Build history of the part. All positions in model axes, mm. A direction names the side the tool comes from. Round coordinates to 2 decimals unless told otherwise and drop trailing zeros. Write each loop counter-clockwise with the first axis right and the second up, starting at its lowest first coordinate (ties: lowest second). Pieces come first, ordered by that corner, then holes.
1) Saw through at B-B (x = -6.35). Write the cut outline in (y, z), plus the area to 3 significant figures.
2) Wall check: probe 1 along Z at (x, y) = (-6, 4); probe 2 along Z at (x, y) = (-33.76, 4); probe 3 along X at (y, z) = (5.5, -13.41). Give the ranges that are in metal, low to high.
3) Saw through at C-C (y = 25). Write the cut outline in (x, z).
4) Flat gauge pins, fed straight in: pin 1 (2 mm diameter, centred on y = 33, z = -23.5, fed in from +X); pin 2 (12 mm diameter, centred on x = -30.5, z = 23, fed in from +Y); pin 3 (1.5 mm diameter, centred on x = 29.5, y = 32, fed in from +Z). Where does each tip first touch, or does it go through?
5) Which spindle directions (+Z, -Z, +X, -X, +Y, -Y) get a long thin tool onto all of the face, cutting with end or side? Do faces 5 (the flat face through (-59, 6, 25.4)), 6 (the flat face through (12.986, 18, 0)), 7 (the flat face through (14.986, 23, 0)), 8 (the flat face through (14.986, 32, 23)). Say none if no direction does.
6) Saw through at A-A (z = 0). Write the cut outline in (x, y).
7) Pull direction X, two halves, no side cores. Call faces 1 (the cylindrical face through (-6.61, 3.5, -65.085)), 2 (the flat face through (51, 18, 25.4)), 3 (the flat face through (-20, 7.1, -1)), 4 (the flat face through (86.36, 23, 0)): +X half, -X half, draft (parallel to the pull), parting line (faces both ways), or undercut.
8) Saw through at D-D (x = 49). Write the cut outline in (y, z), plus the area to 3 significant figures.
from build123d import *

# Parameters (mm, degrees)
SKETCH1_W           = 172.72
SKETCH1_H           = 50.8
BOSS_EXTRUDE1_DEPTH = 12.7
BOSS_EXTRUDE2_DEPTH = 71.374
SKETCH5_W           = 50.8
SKETCH5_H           = 27.94
BOSS_EXTRUDE3_DEPTH = 2
SKETCH6_W           = 50.8
SKETCH6_H           = 15.24
BOSS_EXTRUDE4_DEPTH = 2
CUT_EXTRUDE1_DEPTH  = 51.8
FILLET1_R           = 1
SKETCH8_R           = 12.7
CUT_EXTRUDE2_DEPTH  = 7.1
SKETCH9_R           = 5.9563
BOSS_EXTRUDE5_DEPTH = 7.1
SKETCH10_R          = 1.5
CUT_EXTRUDE3_DEPTH  = 7.1


with BuildPart() as part:
    # Sketch1 → Boss-Extrude1 (new body)
    with BuildSketch(Plane(origin=(0, 0, 0), x_dir=(1, 0, 0), z_dir=(0, 1, 0))):
        Rectangle(SKETCH1_W, SKETCH1_H)
    extrude(amount=BOSS_EXTRUDE1_DEPTH)

    # Sketch4 → Boss-Extrude2 (add)
    with BuildSketch(Plane(origin=(86.36, 0, 0), x_dir=(0, 0, -1), z_dir=(1, 0, 0))):
        with BuildLine():
            Line((-25.4, 12.7), (-25.4, 35.8))
            Line((-25.4, 35.8), (-20.1, 35.8))
            ThreePointArc((-20.1, 35.8), (0, 15.7), (20.1, 35.8))
            Line((20.1, 35.8), (25.4, 35.8))
            Line((25.4, 35.8), (25.4, 12.7))
            Line((25.4, 12.7), (-25.4, 12.7))
        make_face()
    extrude(amount=-BOSS_EXTRUDE2_DEPTH)

    # Sketch5 → Boss-Extrude3 (add)
    with BuildSketch(Plane(origin=(86.36, 0, 0), x_dir=(0, 0, -1), z_dir=(1, 0, 0))):
        with Locations((0, 13.97)):
            Rectangle(SKETCH5_W, SKETCH5_H)
    extrude(amount=BOSS_EXTRUDE3_DEPTH)

    # Sketch6 → Boss-Extrude4 (add)
    with BuildSketch(Plane.ZY.offset(-14.986)):
        with Locations((0, 20.32)):
            Rectangle(SKETCH6_W, SKETCH6_H)
    extrude(amount=BOSS_EXTRUDE4_DEPTH)

    # Sketch7 → Cut-Extrude1 (cut, through all)
    with BuildSketch(Plane.XY.offset(25.4)):
        Polygon((-86.36, 12.7), (-86.36, 11.7), (-54.96, 11.7), (-54.96, 10.1), (-46.45999982, 10.1), (-46.45999982, 7.1), (12.986, 7.1), (12.986, 12.7), align=None)
    extrude(amount=-CUT_EXTRUDE1_DEPTH, mode=Mode.SUBTRACT)

    # Fillet1
    fillet1_edges = [part.edges().sort_by_distance(p)[0] for p in [
        (-46.45999982, 10.1, 0),
    ]]
    fillet(fillet1_edges, radius=FILLET1_R)

    # Sketch8 → Cut-Extrude2 (cut)
    with BuildSketch(Plane.XZ):
        with Locations((-6.35, 0)):
            Circle(SKETCH8_R)
    extrude(amount=-CUT_EXTRUDE2_DEPTH, mode=Mode.SUBTRACT)

    # Sketch9 → Boss-Extrude5 (add)
    with BuildSketch(Plane(origin=(0, 0, 0), x_dir=(1, 0, 0), z_dir=(0, 1, 0))):
        with BuildLine():
            Line((-33.02, 25.4), (-20.875030517, 55.308759963))
            ThreePointArc((-20.875030517, 55.308759963), (-6.35, 65.0875), (8.175030517, 55.308759963))
            Line((8.175030517, 55.308759963), (20.32, 25.4))
            Line((20.32, 25.4), (-33.02, 25.4))
        make_face()
        with Locations((-6.35, 49.41062)):
            Circle(SKETCH9_R, mode=Mode.SUBTRACT)
        with BuildLine():
            Line((20.32, -25.4), (-33.02, -25.4))
            Line((-33.02, -25.4), (-20.875030517, -55.308759963))
            ThreePointArc((-20.875030517, -55.308759963), (-6.35, -65.0875), (8.175030517, -55.308759963))
            Line((8.175030517, -55.308759963), (20.32, -25.4))
        make_face()
        with Locations((-6.35, -49.41062)):
            Circle(SKETCH9_R, mode=Mode.SUBTRACT)
    extrude(amount=BOSS_EXTRUDE5_DEPTH)

    # Sketch10 → Cut-Extrude3 (cut)
    with BuildSketch(Plane(origin=(0, 7.1, 0), x_dir=(1, 0, 0), z_dir=(0, 1, 0))):
        with Locations((-33.75999982, 13.41)):
            Circle(SKETCH10_R)
        with Locations((-33.75999982, -13.31)):
            Circle(SKETCH10_R)
    extrude(amount=-CUT_EXTRUDE3_DEPTH, mode=Mode.SUBTRACT)


solid = part.part
Evaluation:
1. outline: (0, -65.09) - (7.1, -65.09) - (7.1, -55.37) - (0, -55.37) - close; (0, -43.45) - (7.1, -43.45) - (7.1, -12.7) - (0, -12.7) - close; (0, 12.7) - (7.1, 12.7) - (7.1, 43.45) - (0, 43.45) - close; (0, 55.37) - (7.1, 55.37) - (7.1, 65.09) - (0, 65.09) - close
1. area: 575 mm2
2. probe 1: z = -65.08 to -55.36, -43.46 to -12.7, 12.7 to 43.46, 55.36 to 65.08
2. probe 2: z = -25.4 to -14.91, -11.91 to 11.81, 14.81 to 25.4
2. probe 3: x = -86.36 to -35.26, -32.26 to 88.36
3. outline: (12.99, -25.4) - (88.36, -25.4) - (88.36, 25.4) - (12.99, 25.4) - close; hole (14.99, -16.95) - (86.36, -16.95) - (86.36, 16.95) - (14.99, 16.95) - close
4. pin 1: stops at x = 86.36
4. pin 2: stops at y = 7.1
4. pin 3: stops at z = 25.4
5. face 5: +Z, -X, +Y, -Y
5. face 6: +Z, -Z, +Y
5. face 7: +Y
5. face 8: +Z, -Z, -X, +Y
6. outline: (-86.36, 0) - (-19.05, 0) - (-19.05, 7.1) - (-46.46, 7.1) - (-46.46, 9.1) arc R1 ccw to (-47.46, 10.1) - (-54.96, 10.1) - (-54.96, 11.7) - (-86.36, 11.7) - close; (6.35, 0) - (88.36, 0) - (88.36, 27.94) - (86.36, 27.94) - (86.36, 15.7) - (14.99, 15.7) - (14.99, 27.94) - (12.99, 27.94) - (12.99, 7.1) - (6.35, 7.1) - close
7. face 1: parting line
7. face 2: draft
7. face 3: undercut
7. face 4: undercut
8. outline: (0, -25.4) - (35.8, -25.4) - (35.8, -20.1) arc R20.1 cw to (35.8, 20.1) - (35.8, 25.4) - (0, 25.4) - close
8. area: 1,180 mm2
